Verification items for this drawing (mm, ordinates from the low corner). A direction names the side the tool comes from. Give positions to 0.01 mm unless a question says otherwise; leave off trailing zeros. Order: outer loops, then holes, each group sorted by start corner. A loop starts at its lowest first (then second) coordinate and runs counter-clockwise, first axis right, second up.
(1) Access from +Z, -Z, +X, -X, +Y, -Y to the whole of each face (thin tool, end or side, straight path). Record for the marked faces 4 and 5.
(2) Sectioned sample at D-D on x = 4.4. Record the cut outline in (y, z).
(3) Sectioned sample at C-C on z = 2.95. Record the cut outline in (x, y).
(4) Sectioned sample at A-A on y = 0.6. Record the cut outline in (x, z).
(5) Gauge pin test, flat ends, axial feed: pin 1 (1 mm diameter, centred on x = 1, y = 0.5, fed in from +Z); pin 2 (1.5 mm diameter, centred on y = 2.5, z = 1.5, fed in from -X). Record the tip position at first contact, or that the pin passes through.
(6) Scan lines: L1, parallel to Z at x = 1.9, y = 0.2 (1 decimal); L2, parallel to X at y = 2.55, z = 3.8; L3, parallel to X at y = 1.3, z = 1.6. Record each from-to range of solid material in increasing order.
(7) Sectioned sample at B-B on x = 2.75. Record the cut outline in (y, z).
(8) Mould release check, pull along X, two halves, no side actions. Record for the marked faces 1, 2 and 3: pulls with the +X half, pulls with the -X half, needs draft (parallel to the pull), parting line crosses it, or undercut.
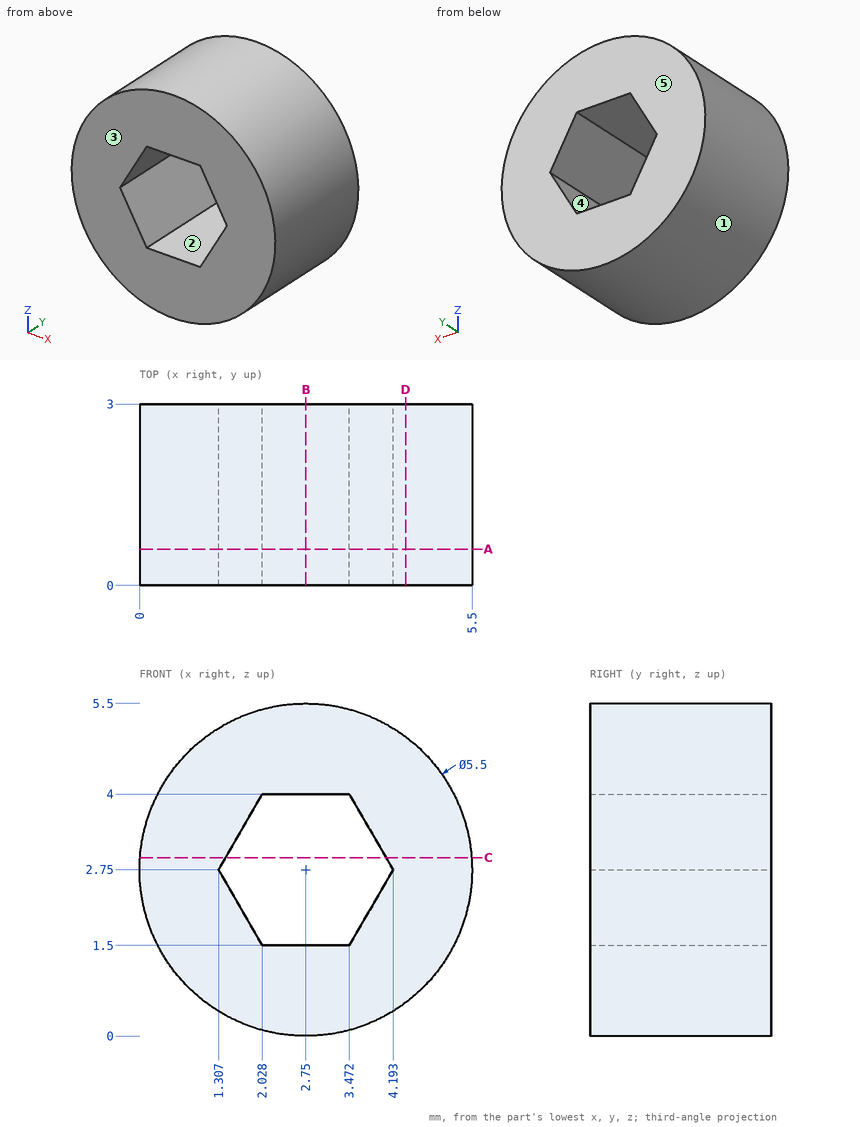
Ans:
1. face 4: +Y, -Y
1. face 5: +Z, -Z, +X, -X, +Y
2. outline: (0, 0.55) - (3, 0.55) - (3, 4.95) - (0, 4.95) - close
3. outline: (0.01, 0) - (1.42, 0) - (1.42, 3) - (0.01, 3) - close; (4.08, 0) - (5.49, 0) - (5.49, 3) - (4.08, 3) - close
4. outline: circle Ø5.5 at (2.75, 2.75); hole (1.31, 2.75) - (2.03, 1.5) - (3.47, 1.5) - (4.19, 2.75) - (3.47, 4) - (2.03, 4) - close
5. pin 1: stops at z = 5.2
5. pin 2: stops at x = 0.05
6. L1: z = 0.1 to 1.7, 3.8 to 5.4
6. L2: x = 0.21 to 1.91, 3.59 to 5.29
6. L3: x = 0.25 to 1.97, 3.53 to 5.25
7. outline: (0, 0) - (3, 0) - (3, 1.5) - (0, 1.5) - close; (0, 4) - (3, 4) - (3, 5.5) - (0, 5.5) - close
8. face 1: parting line crosses it
8. face 2: undercut
8. face 3: needs draft
